Can you work these out from the model? Positions are in its coordinate system, mm. A direction names the side the tool comes from. Give positions to 0.01 mm unless a question says otherwise; leave off trailing zeros. Loops run counter-clockwise (first coordinate to the right, second up) from the corner with the lowest first, then second, coordinate; pieces in that order, holes last. Notation, with made-up numbers: (73, 87.5) - (81, 87.5) arc R26 cw to (81, 102.5) - close; hole circle Ø3 at (-12.75, -11). An arc over 180 degrees is marked (long way). Write item = value, one per line.
from build123d import *

# Parameters (mm, degrees)
BOSS_EXTRUDE1_DEPTH = 20
SKETCH2_W           = 106.8
SKETCH2_H           = 20
BOSS_EXTRUDE2_DEPTH = 5
BOSS_EXTRUDE3_DEPTH = 12.5
SKETCH4_W           = 90.804234884
SKETCH4_H           = 53.3
BOSS_EXTRUDE4_DEPTH = 10
SKETCH7_R           = 2.9
CUT_EXTRUDE3_DEPTH  = 129.904719117
BOSS_EXTRUDE6_START = 53.3
SKETCH8_R           = 2.9
SKETCH8_W           = 10
SKETCH8_H           = 10
BOSS_EXTRUDE6_DEPTH = 53.3
BOSS_EXTRUDE7_DEPTH = 22.5
SKETCH12_R          = 2.9
CUT_EXTRUDE6_DEPTH  = 132.051236585
BOSS_EXTRUDE8_DEPTH = 4


with BuildPart() as part:
    # Sketch1 → Boss-Extrude1 (new body)
    with BuildSketch(Plane.XY):
        Polygon((-2.4, 58.3), (-1.02915952, 25), (-0.02915952, 25), (2.6, 35.023161884), (2.6, 58.3), align=None)
        Polygon((7.6, 58.3), (2.6, 58.3), (2.6, 35.023161884), (7.394168096, 53.3), align=None)
        Polygon((19.7, 58.3), (9.7, 58.3), (11.07084048, 25), (12.07084048, 25), (19.494168096, 53.3), align=None)
        Polygon((31.8, 58.3), (21.8, 58.3), (23.17084048, 25), (24.17084048, 25), (31.594168096, 53.3), align=None)
        Polygon((43.9, 58.3), (33.9, 58.3), (35.27084048, 25), (36.27084048, 25), (43.694168096, 53.3), align=None)
        Polygon((56, 58.3), (46, 58.3), (47.37084048, 25), (48.37084048, 25), (55.794168096, 53.3), align=None)
        Polygon((68.1, 58.3), (58.1, 58.3), (59.47084048, 25), (60.47084048, 25), (67.894168096, 53.3), align=None)
        Polygon((80.2, 58.3), (70.2, 58.3), (71.57084048, 25), (72.57084048, 25), (79.994168096, 53.3), align=None)
        Polygon((92.3, 58.3), (82.3, 58.3), (83.67084048, 25), (84.67084048, 25), (92.094168096, 53.3), align=None)
        Polygon((104.4, 58.3), (94.4, 58.3), (95.77084048, 25), (96.77084048, 25), (104.194168096, 53.3), align=None)
        Polygon((84.67084048, 25), (83.67084048, 25), (84.7, 0), (89.9, 0), (90.105831904, 5), align=None)
        Polygon((72.57084048, 25), (71.57084048, 25), (72.6, 0), (77.8, 0), (78.005831904, 5), align=None)
        Polygon((60.47084048, 25), (59.47084048, 25), (60.5, 0), (65.7, 0), (65.905831904, 5), align=None)
        Polygon((48.37084048, 25), (47.37084048, 25), (48.4, 0), (53.6, 0), (53.805831904, 5), align=None)
        Polygon((36.27084048, 25), (35.27084048, 25), (36.3, 0), (41.5, 0), (41.705831904, 5), align=None)
        Polygon((24.17084048, 25), (23.17084048, 25), (24.2, 0), (29.4, 0), (29.605831904, 5), align=None)
        Polygon((12.07084048, 25), (11.07084048, 25), (12.1, 0), (17.3, 0), (17.505831904, 5), align=None)
    extrude(amount=BOSS_EXTRUDE1_DEPTH)

    # Sketch2 → Boss-Extrude2 (add)
    with BuildSketch(Plane(origin=(0, 58.3, 0), x_dir=(1, 0, 0), z_dir=(0, 1, 0))):
        with Locations((51, -10)):
            Rectangle(SKETCH2_W, SKETCH2_H)
    extrude(amount=BOSS_EXTRUDE2_DEPTH)

    # Sketch3 → Boss-Extrude3 (add)
    with BuildSketch(Plane.XY.offset(20)):
        Polygon((109.404234884, 63.3), (107.004234884, 5), (-5, 5), (-7.4, 63.3), align=None)
    extrude(amount=BOSS_EXTRUDE3_DEPTH)

    # Sketch4 → Boss-Extrude4 (add)
    with BuildSketch(Plane.XY.offset(32.5)):
        Polygon((-5, 5), (107.004234884, 5), (107.210066788, 10), (106.404234884, 10), (96.404234884, 10), (5.6, 10), (-4.4, 10), (-5.205831904, 10), align=None)
        Polygon((-7.4, 63.3), (-5.205831904, 10), (-4.4, 10), (-4.4, 63.3), align=None)
        Polygon((107.210066788, 10), (109.404234884, 63.3), (106.404234884, 63.3), (106.404234884, 10), align=None)
        with Locations((51.002117442, 36.65)):
            Rectangle(SKETCH4_W, SKETCH4_H)
    extrude(amount=BOSS_EXTRUDE4_DEPTH)

    # Sketch7 → Cut-Extrude3 (cut, through all)
    with BuildSketch(Plane(origin=(0, 10, 0), x_dir=(1, 0, 0), z_dir=(0, 1, 0))):
        with Locations(Location((101.404234884, -29.5, 0), (0, 0, 180))):
            Circle(SKETCH7_R)
        with Locations(Location((0.6, -29.5, 0), (0, 0, 180))):
            Circle(SKETCH7_R)
    extrude(amount=-CUT_EXTRUDE3_DEPTH, mode=Mode.SUBTRACT)

    # Sketch8 → Boss-Extrude6 (add)
    with BuildSketch(Plane(origin=(0, 10, 0), x_dir=(1, 0, 0), z_dir=(0, 1, 0)).offset(BOSS_EXTRUDE6_START)):
        with Locations(Location((101.404234884, -29.5, 0), (0, 0, 180))):
            Circle(SKETCH8_R)
        with Locations(Location((0.6, -29.5, 0), (0, 0, 180))):
            Circle(SKETCH8_R)
        with Locations((101.404234884, -37.5)):
            Rectangle(SKETCH8_W, SKETCH8_H)
        with Locations((0.6, -37.5)):
            Rectangle(SKETCH8_W, SKETCH8_H)
    extrude(amount=-BOSS_EXTRUDE6_DEPTH)

    # Sketch10 → Boss-Extrude7 (add)
    with BuildSketch(Plane.XY.offset(20)):
        Polygon((-5, 5), (-4.794168096, 0), (106.79840298, 0), (107.004234884, 5), align=None)
    extrude(amount=BOSS_EXTRUDE7_DEPTH)

    # Sketch12 → Cut-Extrude6 (cut, through all)
    with BuildSketch(Plane(origin=(0, 5, 0), x_dir=(1, 0, 0), z_dir=(0, 1, 0))):
        with Locations(Location((101.404234884, -29.5, 0), (0, 0, 180))):
            Circle(SKETCH12_R)
        with Locations(Location((0.6, -29.5, 0), (0, 0, 180))):
            Circle(SKETCH12_R)
    extrude(amount=-CUT_EXTRUDE6_DEPTH, mode=Mode.SUBTRACT)

    # Sketch13 → Boss-Extrude8 (add)
    # profile 1 of 2: a face of its own
    with BuildSketch(Plane.XY.offset(42.5)):
        Polygon((108.992571076, 53.3), (107.210066788, 10), (117.210066788, 10), (117.210066788, 53.3), align=None)
        with BuildLine():
            Line((110.313406273, 15.041157663), (110.998826513, 48.341157663))
            ThreePointArc((110.998826513, 48.341157663), (113.039560643, 50.299576467), (114.997979447, 48.258842337))
            Line((114.997979447, 48.258842337), (114.312559207, 14.958842337))
            ThreePointArc((114.312559207, 14.958842337), (112.271825077, 13.000423533), (110.313406273, 15.041157663))
        make_face(mode=Mode.SUBTRACT)
    # profile 2 of 2: a face of its own
    with BuildSketch(Plane.XY.offset(42.5)):
        Polygon((-15.205831904, 10), (-15.205831904, 53.3), (-6.988336192, 53.3), (-5.205831904, 10), align=None)
        with BuildLine():
            Line((-8.309171389, 15.041157663), (-8.994591629, 48.341157663))
            ThreePointArc((-8.994591629, 48.341157663), (-11.035325759, 50.299576467), (-12.993744563, 48.258842337))
            Line((-12.993744563, 48.258842337), (-12.308324323, 14.958842337))
            ThreePointArc((-12.308324323, 14.958842337), (-10.267590193, 13.000423533), (-8.309171389, 15.041157663))
        make_face(mode=Mode.SUBTRACT)
    extrude(amount=-BOSS_EXTRUDE8_DEPTH)


solid = part.part
Q1. I need wall thicknesses on L1, parallel to X at y = 3, z = 29; L2, parallel to X at y = 4, z = 29; L3, parallel to Z at x = 0.6, y = 3.5. Which ranges of each line are inside material? Lowest first, please.
Output:
L1 = -4.92 to -2.26, 3.46 to 98.55, 104.26 to 106.92
L2 = -4.96 to -2.26, 3.46 to 98.55, 104.26 to 106.96
L3 = 20 to 26.6, 32.4 to 42.5
Q2. Which directions (+Z, -Z, +X, -X, +Y, -Y) give clear straight access to the entire face, cutting with the end or side of a thin tool? Please do faces 1 (the flat face through (2, 25, 20)), 2 (the flat face through (27.83, 38.95, 9.86)), 3 (the cylindrical face through (113, 50.3, 40.5)), 4 (the flat face through (112, 10, 41)).
Output:
face_1 = -Z, -Y
face_2 = -Z
face_3 = +Z, -Z
face_4 = +Z, -Z, +X, -Y
Q3. Imagine slicing it at B-B, the plane y = 37. Give the number of separate pieces and of enclosed holes in the cut face, then the cut area to 3 significant figures.
Output:
separate_pieces = 3
enclosed_holes = 0
area = 3,450 mm2
Q4. We'd pull the mould along Y, two halves only. Please class faces 5 (the flat face through (55.896, 55.765, 9.86)), 6 (the flat face through (15.73, 38.95, 9.86)), 7 (the flat face through (50, 38, 0)), 8 (the flat face through (76.23, 38.95, 9.86)): released by +Y, released by -Y, zero draft, split by the parting line, or undercut.
Output:
face_5 = released by -Y
face_6 = undercut
face_7 = zero draft
face_8 = undercut
Q5. Imagine slicing it at C-C, the plane z = 22.5. Write out the boundary of the cut face in (x, y).
Output:
outline = (-7.4, 63.3) - (-4.79, 0) - (106.8, 0) - (109.4, 63.3) - close
Q6. Imagine slicing it at A-A, the plane z = 29.5. Write out the boundary of the cut face in (x, y).
Output:
outline = (-7.4, 63.3) - (-4.79, 0) - (-2.3, 0) - (-2.3, 10) - (3.5, 10) - (3.5, 0) - (98.5, 0) - (98.5, 10) - (104.3, 10) - (104.3, 0) - (106.8, 0) - (109.4, 63.3) - close
Q7. For pin 1 (1.7 mm diameter, centred on x = 0.5, z = 30, fed in from -Y); pin 2 (10 mm diameter, centred on y = 31.5, z = 28.5, fed in from +X); pin 3 (11 mm diameter, centred on x = -8.5, y = 21.5, fed in from -Z); pin 4 (3.5 mm diameter, centred on x = 52, y = 36, fed in from -Z), each with a flat end and sliding along its axis, tell me the tip position at first contact or that it passes through.
Output:
pin_1 = 10
pin_2 = 108.3
pin_3 = 20
pin_4 = 0
